Geometry: final body of the model. Coordinates: model frame, mm. Coordinates: 2 decimals unless noted, no trailing zeros. Loops run counter-clockwise (first coordinate to the right, second up) from the corner with the lowest first, then second, coordinate; pieces in that order, holes last. Notation, with made-up numbers: (-20.75, -6.5) -> (-7.75, -6.5) arc R31 ccw to (-7.75, 31.5) -> close; hole circle Ø2 at (-2.5, 50). An arc over 180 degrees is marked (long way). One line per item, written item: value. Start each with the question number.
Item 1: Contact query for a flat-ended pin moving along its axis: pin 1 Ø4 at (x, y) = (-59.49, 7.83) entering from +Z. Output: stop coordinate, or through.
Item 2: Section query B-B on z = 0.4. Give the number of separate pieces and of enclosed holes in the cut face, then the cut area to 3 significant figures.
Item 3: Ray query, probe 1 along X at (y, z) = (42, -0.2); probe 2 along X at (y, z) = (53, 0.05) (1 decimal); probe 3 along X at (y, z) = (25, -0.65). Return the intervals inside material, ascending. Write a range as from..to.
Item 4: Section query C-C on x = -52. Return loops of the section in (y, z).
Item 5: Section query A-A on x = 0. Return loops of the section in (y, z), then the cut area to 3 significant figures.
from build123d import *

# Parameters (mm, degrees)
BOSS_EXTRUDE1_DEPTH            = 0.762
F_4_CLEARANCE_HOLE1_AT_2_COUNT = 2
F_4_CLEARANCE_HOLE1_AT_2_PITCH = 13
CIRPATTERN1_COUNT              = 4
CIRPATTERN1_ANGLE              = 165
CUT_EXTRUDE1_DEPTH             = 2.524


with BuildPart() as part:
    # Sketch1 → Boss-Extrude1 (new body, symmetric)
    with BuildSketch(Plane.XY):
        with BuildLine():
            Line((-63.386197236, 3.8), (-36.804347569, 3.8))
            ThreePointArc((-36.804347569, 3.8), (0, 37), (36.804347569, 3.8))
            Line((36.804347569, 3.8), (63.386197236, 3.8))
            ThreePointArc((63.386197236, 3.8), (0, 63.5), (-63.386197236, 3.8))
        make_face()
    extrude(amount=BOSS_EXTRUDE1_DEPTH, both=True)

    # Sketch2 → #4 Clearance Hole1 (revolve, cut)
    with BuildSketch(Plane(origin=(-59.486691682, 7.831571533, 0.762), x_dir=(0, -1, 0), z_dir=(1, 0, 0))):
        Polygon((0, 0), (0, 136.775187864), (1.4732, 135.89), (1.4732, 0), align=None)
    f_4_clearance_hole1 = revolve(axis=Axis((-59.486691682, 7.831571533, 7.112), (0, 0, -1)), mode=Mode.SUBTRACT)

    # #4 Clearance Hole1 at 2: #4 Clearance Hole1 ×2
    with Locations(*[Vector(0.991444861, -0.130526192, 0) * (i * F_4_CLEARANCE_HOLE1_AT_2_PITCH) for i in range(1, F_4_CLEARANCE_HOLE1_AT_2_COUNT)]):
        add(f_4_clearance_hole1, mode=Mode.SUBTRACT)

    # CirPattern1: #4 Clearance Hole1 ×4 about axis
    cirpattern1_axis = Axis((0, 0, 0), (0, 0, -1))
    for i in range(1, CIRPATTERN1_COUNT):
        add(f_4_clearance_hole1.rotate(cirpattern1_axis, i * CIRPATTERN1_ANGLE / (CIRPATTERN1_COUNT - 1)), mode=Mode.SUBTRACT)

    # CirPattern1 copy 1 sketch → CirPattern1 copy 1 (revolve, cut)
    with BuildSketch(Plane(origin=(-21.702184822, 41.689509159, 0.762), x_dir=(-0.819152044, -0.573576436, 0), z_dir=(0.573576436, -0.819152044, 0))):
        Polygon((0, 0), (0, 136.775187864), (1.4732, 135.89), (1.4732, 0), align=None)
    revolve(axis=Axis((-21.702184822, 41.689509159, 7.112), (0, 0, -1)), mode=Mode.SUBTRACT)

    # CirPattern1 copy 2 sketch → CirPattern1 copy 2 (revolve, cut)
    with BuildSketch(Plane(origin=(21.702184822, 41.689509159, 0.762), x_dir=(-0.939692621, 0.342020143, 0), z_dir=(-0.342020143, -0.939692621, 0))):
        Polygon((0, 0), (0, 136.775187864), (1.4732, 135.89), (1.4732, 0), align=None)
    revolve(axis=Axis((21.702184822, 41.689509159, 7.112), (0, 0, -1)), mode=Mode.SUBTRACT)

    # CirPattern1 copy 3 sketch → CirPattern1 copy 3 (revolve, cut)
    with BuildSketch(Plane(origin=(46.597908485, 6.134731034, 0.762), x_dir=(-0.258819045, 0.965925826, 0), z_dir=(-0.965925826, -0.258819045, 0))):
        Polygon((0, 0), (0, 136.775187864), (1.4732, 135.89), (1.4732, 0), align=None)
    revolve(axis=Axis((46.597908485, 6.134731034, 7.112), (0, 0, -1)), mode=Mode.SUBTRACT)

    # Sketch4 → Cut-Extrude1 (cut, through all)
    with BuildSketch(Plane.XY.offset(0.762)):
        with BuildLine():
            Line((-4.5, 55), (4.5, 55))
            ThreePointArc((4.5, 55), (6.5, 53), (4.5, 51))
            Line((4.5, 51), (-4.5, 51))
            ThreePointArc((-4.5, 51), (-6.5, 53), (-4.5, 55))
        make_face()
    extrude(amount=-CUT_EXTRUDE1_DEPTH, mode=Mode.SUBTRACT)


solid = part.part
Reply:
1. pin 1: stops at z = 0.76
2. separate pieces: 1
2. enclosed holes: 9
2. area: 3,880 mm²
3. probe 1: x = -47.63..-23.14, -20.26..20.26, 23.14..47.63
3. probe 2: x = -35..-29.2, -26.2..-6.5, 6.5..26.2, 29.2..35
3. probe 3: x = -58.37..-27.28, 27.28..58.37
4. outline: (3.8, -0.76) -> (36.45, -0.76) -> (36.45, 0.76) -> (3.8, 0.76) -> close
5. outline: (37, -0.76) -> (51, -0.76) -> (51, 0.76) -> (37, 0.76) -> close; (55, -0.76) -> (63.5, -0.76) -> (63.5, 0.76) -> (55, 0.76) -> close
5. area: 34.3 mm²
